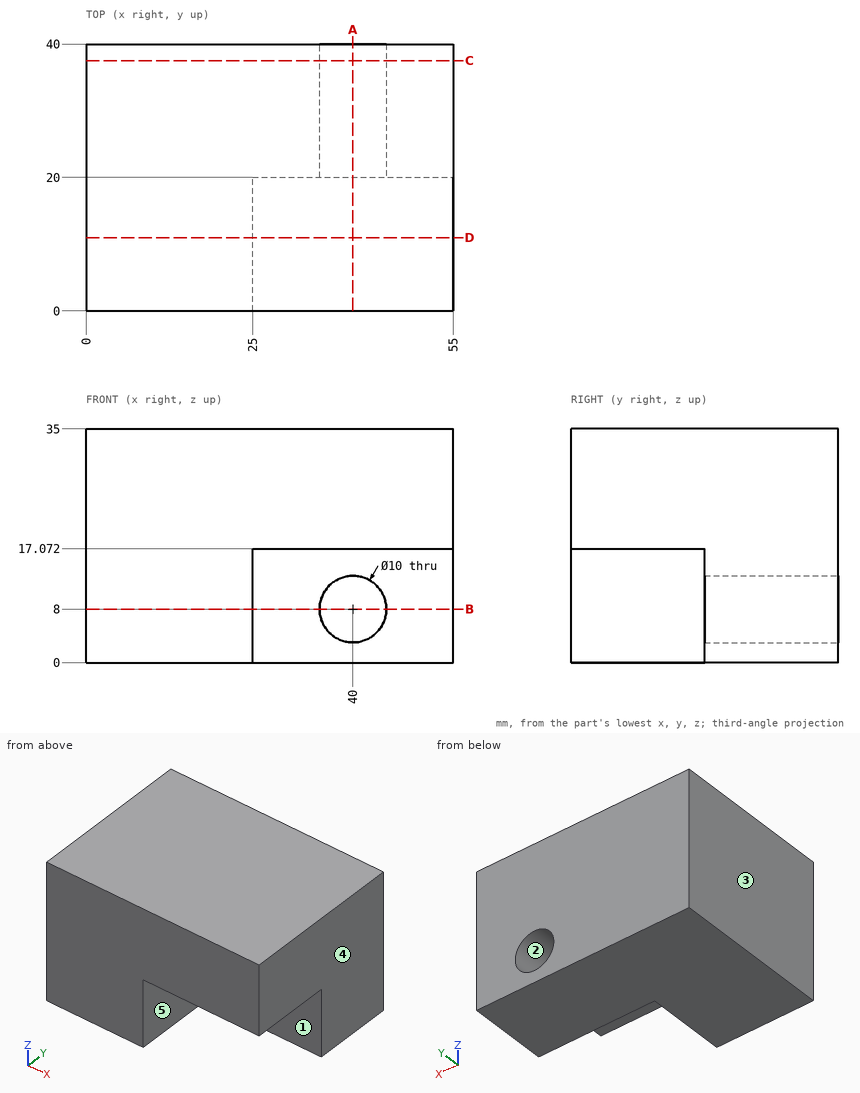
Check sheet for the drawn part. Datum: minimum x, y, z corner. Units: mm. A direction names the side the tool comes from. Round coordinates to 2 decimals unless told otherwise and drop trailing zeros. Loops run counter-clockwise (first coordinate to the right, second up) from the corner with the lowest first, then second, coordinate; pieces in that order, holes last. Notation, with made-up numbers: (48.25, -29.75) - (63.25, -29.75) arc R16 cw to (63.25, -6.75) - close; hole circle Ø11 at (-36.75, 64.5). An arc over 180 degrees is marked (long way). Write item = value, one per line. Start each with the question number.
1. Depth check by flat-ended pin: pin 1 (16 mm diameter, centred on x = 46, y = 10.5, fed in from -Z); pin 2 (9 mm diameter, centred on x = 40, z = 8, fed in from -Y); pin 3 (5 mm diameter, centred on x = 38, z = 12, fed in from -Y). Enter the tip coordinate at first touch or a pass-through.
2. Thickness scan on line 1 (Z direction, x = 40, y = 35.75); line 2 (Y direction, x = 51, z = 8); line 3 (X direction, y = 3, z = 16). Record the ranges inside material, lowest first.
3. Section check D-D on y = 11. Enter the section's corners in (x, z), then the cut area to 3 significant figures.
4. Mould release check, pull along X, two halves, no side actions. Record for the marked faces 1, 2 and 3: released by +X, released by -X, zero draft, split by the parting line, or undercut.
5. Section check B-B on z = 8. Enter the section's corners in (x, y), then the cut area to 3 significant figures.
6. Section check C-C on y = 37.5. Enter the section's corners in (x, z), then the cut area to 3 significant figures.
7. Set-up check for the marked faces 4 and 5: record each of +Z, -Z, +X, -X, +Y, -Y from which the full face is reachable in a straight line by a thin tool's end or side.
8. Section check A-A on x = 40. Enter the section's corners in (y, z), then the cut area to 3 significant figures.
Working result:
q1.pin_1 = 17.07
q1.pin_2 = through
q1.pin_3 = 20
q2.line_1 = 0 to 3, 13 to 35
q2.line_2 = 20 to 40
q2.line_3 = 0 to 25
q3.outline = (0, 0) - (25, 0) - (25, 17.07) - (55, 17.07) - (55, 35) - (0, 35) - close
q3.area = 1,410 mm^2
q4.face_1 = zero draft
q4.face_2 = undercut
q4.face_3 = released by -X
q5.outline = (0, 0) - (25, 0) - (25, 20) - (35, 20) - (35, 40) - (0, 40) - close; (45, 20) - (55, 20) - (55, 40) - (45, 40) - close
q5.area = 1,400 mm^2
q6.outline = (0, 0) - (55, 0) - (55, 35) - (0, 35) - close; hole circle Ø10 at (40, 8)
q6.area = 1,850 mm^2
q7.face_4 = +Z, -Z, +X, +Y, -Y
q7.face_5 = -Z, +X, -Y
q8.outline = (0, 17.07) - (20, 17.07) - (20, 13) - (40, 13) - (40, 35) - (0, 35) - close; (20, 0) - (40, 0) - (40, 3) - (20, 3) - close
q8.area = 859 mm^2
